Can you work these out from the drawing? Everything is in mm from the part's minimum corner. A direction names the side the tool comes from. Coordinates: 2 decimals unless noted, no trailing zeros. Loops run counter-clockwise (first coordinate to the right, second up) from the corner with the lowest first, then second, coordinate; pieces in that order, holes last.
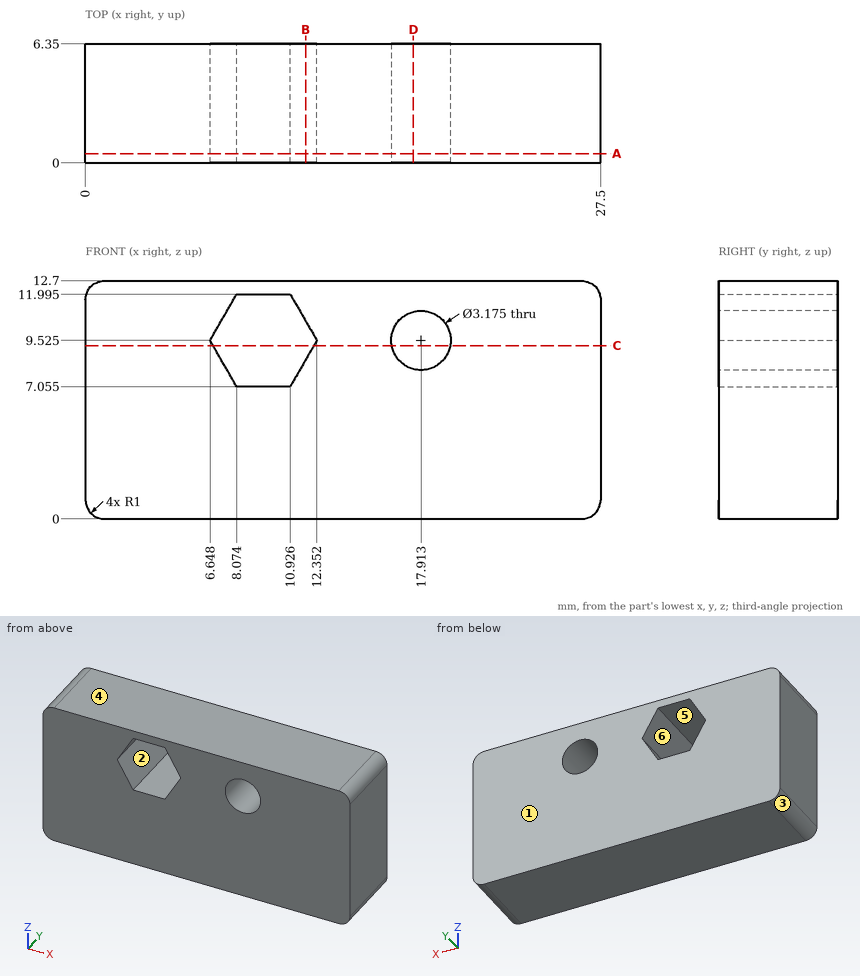
Item 1: Suppose I cut it at B-B, the plane x = 11.75. Please give me the cut outline in (y, z).
Results are:
outline: (0, 0) - (6.35, 0) - (6.35, 8.48) - (0, 8.48) - close; (0, 10.57) - (6.35, 10.57) - (6.35, 12.7) - (0, 12.7) - close
Item 2: On a 3-axis mill with a long thin cutter (end or side, diameter ignored), from which of +Z, -Z, +X, -X, +Y, -Y can I reach the whole of each face in a straight line? I mean the marked faces 1 and 2. Say none if no direction works.
Results are:
face 1: +Z, -Z, +X, -X, +Y
face 2: +Y, -Y
Item 3: Suppose I cut it at A-A, the plane y = 0.5. Please give me the cut outline in (x, z) (1 decimal), plus the area to 3 significant figures.
Results are:
outline: (0, 1) arc R1 ccw to (1, 0) - (26.5, 0) arc R1 ccw to (27.5, 1) - (27.5, 11.7) arc R1 ccw to (26.5, 12.7) - (1, 12.7) arc R1 ccw to (0, 11.7) - close; hole (6.6, 9.5) - (8.1, 7.1) - (10.9, 7.1) - (12.4, 9.5) - (10.9, 12) - (8.1, 12) - close; hole circle Ø3.2 at (17.9, 9.5)
area: 319 mm2
Item 4: I need wall thicknesses on line 1 along Z through (x, y) = (9.5, 4) (1 decimal); line 2 along X through (y, z) = (4.5, 8.75) (1 decimal); line 3 along X through (y, z) = (1, 10.5) (1 decimal). Which ranges of each line are inside material? Lowest first, please.
Results are:
line 1: z = 0 to 7.1, 12 to 12.7
line 2: x = 0 to 7.1, 11.9 to 16.5, 19.3 to 27.5
line 3: x = 0 to 7.2, 11.8 to 16.7, 19.2 to 27.5
Item 5: Suppose I cut it at C-C, the plane z = 9.25. Count the separate pieces of the cut face and the enclosed holes in it.
Results are:
separate pieces: 3
enclosed holes: 0
Item 6: Suppose I cut it at D-D, the plane x = 17.5. Please give me the cut outline in (y, z).
Results are:
outline: (0, 0) - (6.35, 0) - (6.35, 7.99) - (0, 7.99) - close; (0, 11.06) - (6.35, 11.06) - (6.35, 12.7) - (0, 12.7) - close
Item 7: We'd pull the mould along X, two halves only. Please class the marked faces 3, 4, 5 and 6: +X half, -X half, draft (parallel to the pull), parting line (faces both ways), or undercut.
Results are:
face 3: -X half
face 4: draft
face 5: undercut
face 6: undercut
